```python
from build123d import *

# Parameters (mm, degrees)
F0_R     = 1.6
F1_DEPTH = 3


# Not quite as in the source:
# - ends of sketch curves that miss each other by under 0.0002 mm in the source are joined


with BuildPart() as f1:
    # F0 (on Front) → F1 (new body)
    with BuildSketch(Plane.XZ):
        with BuildLine():
            ThreePointArc((-10.6282638986, 3.1898001668), (-12.4668430477, 5.2626032061), (-13.8612036619, 7.6568972993))
            ThreePointArc((-13.8612036619, 7.6568972993), (-18.9011019651, 9.7424118848), (-21.335831, 4.861629))
            Line((-21.335831, 4.861629), (-16.648169, -10.991964))
            Line((-16.648169, -10.991964), (-16.648169, -13.674139))
            Line((-16.648169, -13.674139), (-14.092108, -13.6741314818))
            ThreePointArc((-14.092108, -13.6741314818), (-13.8399289655, -13.6065603025), (-13.6553211195, -13.4219524128))
            ThreePointArc((-13.6553211195, -13.4219524128), (-12.8619020996, -13.3175012704), (-12.9663588806, -14.1109235459))
            ThreePointArc((-12.9663588806, -14.1109235459), (-13.1509652395, -14.295530508), (-13.2185364188, -14.5477095425))
            Line((-13.2185364188, -14.5477095425), (-13.2185364188, -16.174139))
            ThreePointArc((-13.2185364188, -16.174139), (-13.0720898094, -16.5276923906), (-12.7185364188, -16.674139))
            Line((-12.7185364188, -16.674139), (-7.66624, -16.674139))
            ThreePointArc((-7.66624, -16.674139), (-7.3126880282, -16.5276923906), (-7.1662414188, -16.174139))
            Line((-7.1662414188, -16.174139), (-7.1662414188, -14.547714))
            ThreePointArc((-7.1662414188, -14.547714), (-7.2338128147, -14.2955345905), (-7.4184212378, -14.1109266865))
            ThreePointArc((-7.4184212378, -14.1109266865), (-7.522878567, -13.3175058971), (-6.7294565149, -13.4219591693))
            ThreePointArc((-6.7294565149, -13.4219591693), (-6.5448489948, -13.6065653787), (-6.2926709268, -13.674136))
            Line((-6.2926709268, -13.674136), (-1.113951, -13.674139))
            Line((-1.113951, -13.674139), (-1.113951, -10.64802))
            Line((-1.113951, -10.64802), (-2.400059, -10.64802))
            Line((-2.400059, -10.64802), (-2.400059, -6.613128))
            Line((-2.400059, -6.613128), (-1.113951, -6.613128))
            Line((-1.113951, -6.613128), (-1.113951, -3.174139))
            Line((-1.113951, -3.174139), (2.113951, -3.174141))
            Line((2.113951, -3.174141), (2.113951, -6.613128))
            Line((2.113951, -6.613128), (3.400058, -6.613128))
            Line((3.400058, -6.613128), (3.400059, -10.64802))
            Line((3.400059, -10.64802), (2.113951, -10.64802))
            Line((2.113951, -10.64802), (2.113951, -13.674139))
            Line((2.113951, -13.674139), (7.292668, -13.6741438699))
            ThreePointArc((7.292668, -13.6741438699), (7.5448470345, -13.6065678207), (7.7294548805, -13.421959931))
            ThreePointArc((7.7294548805, -13.421959931), (8.5228769619, -13.3175030381), (8.418420181, -14.1109253135))
            ThreePointArc((8.418420181, -14.1109253135), (8.2338115208, -14.295533374), (8.16624, -14.547713))
            Line((8.16624, -14.547713), (8.1662414188, -16.174139))
            ThreePointArc((8.1662414188, -16.174139), (8.3126866094, -16.5276923906), (8.66624, -16.674139))
            Line((8.66624, -16.674139), (13.718535, -16.674139))
            ThreePointArc((13.718535, -16.674139), (14.0720883906, -16.5276923906), (14.218535, -16.174139))
            Line((14.218535, -16.174139), (14.2185364188, -14.547713))
            ThreePointArc((14.2185364188, -14.547713), (14.1509638207, -14.2955339655), (13.966355931, -14.1109261195))
            ThreePointArc((13.966355931, -14.1109261195), (13.8618988613, -13.3175032148), (14.6553213135, -13.421959819))
            ThreePointArc((14.6553213135, -13.421959819), (14.8399289655, -13.6065678207), (15.092108, -13.674139))
            Line((15.092108, -13.674139), (17.648169, -13.6741498688))
            Line((17.648169, -13.6741498688), (17.648169, -10.991964))
            ThreePointArc((17.648169, -10.991964), (17.6480727307, -10.9478940797), (17.6477839247, -10.9038250007))
            Line((17.6477839247, -10.9038250007), (17.648169, -10.904063))
            ThreePointArc((17.648169, -10.904063), (21.1804529898, 1.0136018582), (20.7834599948, 13.437375999))
            ThreePointArc((20.7834599948, 13.437375999), (16.5617773272, 16.6632341642), (12.8608694009, 12.8511420265))
            ThreePointArc((12.8608694009, 12.8511420265), (12.4649591094, 10.1088544895), (11.5367438755, 7.4982410587))
            ThreePointArc((11.5367438755, 7.4982410587), (10.2794941976, 6.4290215203), (8.6465971955, 6.6689263042))
            ThreePointArc((8.6465971955, 6.6689263042), (-0.1307148674, 8.353355038), (-7.6378988754, 3.5035408071))
            ThreePointArc((-7.6378988754, 3.5035408071), (-9.062025187, 2.6694105221), (-10.6282638986, 3.1898001668))
        make_face()
        with Locations((-17.5000000032, 5.995824999)):
            Circle(F0_R, mode=Mode.SUBTRACT)
        with BuildLine():
            ThreePointArc((18.4275548403, 12.979433969), (19.0999998798, 5.9958249766), (18.4275548403, -0.9877840157))
            ThreePointArc((18.4275548491, -0.9877839707), (16.5516572505, -2.2530936185), (15.2863477145, -0.3771959445))
            ThreePointArc((15.2863477057, -0.3771959895), (15.8999998798, 5.9958244858), (15.286347893, 12.3688449792))
            ThreePointArc((15.286347905, 12.3688449179), (16.5516567719, 14.2447434618), (18.4275548522, 12.9794339076))
        make_face(mode=Mode.SUBTRACT)
    extrude(amount=F1_DEPTH)


solid = f1.part
```
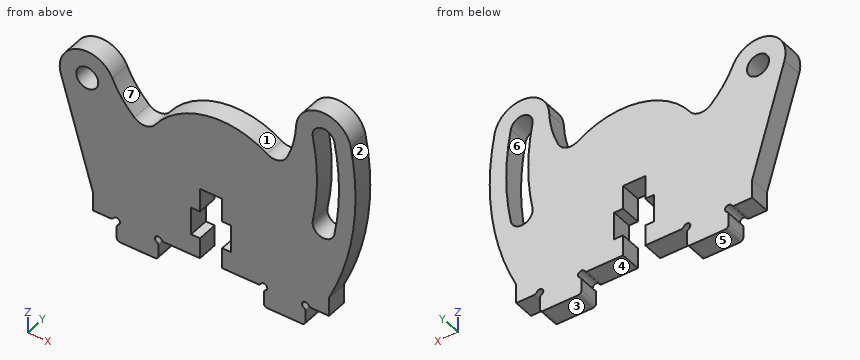
Could you check a few things on this model? Use its own coordinates, in mm. Face numbers are marked on the shaded views. A direction names the side the tool comes from. Give positions to 0.01 mm unless a question says otherwise; leave off trailing zeros. Order: outer loops, then holes, each group sorted by start corner. A loop starts at its lowest first (then second) coordinate and runs counter-clockwise, first axis right, second up.
Q1. Suppose I cut it at A-A, the plane x = -17.5. Write out the boundary of the cut face in (y, z).
Q2. We'd pull the mould along X, two halves only. Please class the marked faces 1, 2 and 3: +X half, -X half, draft (parallel to the pull), parting line (faces both ways), or undercut.
Q3. Suppose I cut it at B-B, the plane y = -0.8. Count the separate pieces of the cut face and the enclosed holes in it, and give its area (3 significant figures).
Q4. For the marked faces 4, 5, 6 and 7, which set-ups out of +Z, -Z, +X, -X, +Y, -Y let a thin tool reach every point of the face, with its end or its side?
Q5. If I drill on line 1 along X through (y, z) = (-1.6, 7); line 2 along X through (y, z) = (-0.9, -13.5); line 3 along X through (y, z) = (-1.55, -12.5), over which ranges is the centre line in solid material (lowest first)?
Q6. I'm going to push flat-ended pins straight in: P1, Ø1.3, axis at y = -1, z = -15.5, coming from the -X side; P2, Ø1.3, axis at y = -1.5, z = -12.5, coming from the -X side; P3, Ø1.3, axis at x = 16.5, y = -1, coming from the -Z side; P4, Ø4, axis at x = -7, z = -8.5, coming from the +Y side. Where does each tip first touch, or does it pass through?
Solution:
1. outline: (-3, -8.11) - (0, -8.11) - (0, 4.4) - (-3, 4.4) - close; (-3, 7.6) - (0, 7.6) - (0, 10) - (-3, 10) - close
2. face 1: undercut
2. face 2: +X half
2. face 3: draft
3. separate pieces: 1
3. enclosed holes: 2
3. area: 815 mm2
4. face 4: -Z, +Y, -Y
4. face 5: -Z, +X, -X, +Y, -Y
4. face 6: +Y, -Y
4. face 7: +Z, +Y, -Y
5. line 1: x = -21.37 to -18.75, -16.25 to -13.54, -3.78 to 8.1, 11.2 to 15.88, 19.09 to 21.49
5. line 2: x = -16.65 to -13.71, -12.75 to -7.64, -6.67 to -1.11, 2.11 to 7.67, 8.64 to 13.75, 14.71 to 17.65
5. line 3: x = -16.65 to -1.11, 2.11 to 17.65
6. P1: stops at x = -13.22
6. P2: stops at x = -16.65
6. P3: stops at z = -13.67
6. P4: stops at y = 0
